from build123d import *
from build123d.topology import SkipClean

# Parameters (mm, degrees)
SKETCH1_W                                       = 111.76
SKETCH1_H                                       = 76.2
BOSS_EXTRUDE1_DEPTH                             = 1.905
FILLET1_R                                       = 2.54
M3_CLEARANCE_HOLE4_D                            = 3.4
CSK_FOR_M3_FLAT_HEAD_MACHINE_SCREW1_D           = 3.4
CSK_FOR_M3_FLAT_HEAD_MACHINE_SCREW1_CSINK_D     = 6.3
CSK_FOR_M3_FLAT_HEAD_MACHINE_SCREW1_CSINK_ANGLE = 90
CSK_FOR_M3_FLAT_HEAD_MACHINE_SCREW2_D           = 3.4
CSK_FOR_M3_FLAT_HEAD_MACHINE_SCREW2_CSINK_D     = 6.3
CSK_FOR_M3_FLAT_HEAD_MACHINE_SCREW2_CSINK_ANGLE = 90
BOSS_EXTRUDE2_START                             = -3.81
SKETCH23_R                                      = 3.15
SKETCH23_R_2                                    = 1.7
BOSS_EXTRUDE2_DEPTH                             = 3.81
SKETCH12_W                                      = 28.355545758
SKETCH12_H                                      = 25.387795591
CUT_EXTRUDE1_DEPTH                              = 68.739947594
M3_CLEARANCE_HOLE1_AT_2_COUNT                   = 2
M3_CLEARANCE_HOLE1_AT_2_PITCH                   = 22.606
FILLET2_R                                       = 2.54


with BuildPart() as part:
    # Sketch1 → Boss-Extrude1 (new, symmetric)
    with BuildSketch(Plane(origin=(0, 0, 0), x_dir=(1, 0, 0), z_dir=(0, 1, 0))):
        Rectangle(SKETCH1_W, SKETCH1_H)
    extrude(amount=BOSS_EXTRUDE1_DEPTH, both=True)

    # Fillet1
    fillet1_edges = [part.edges().sort_by_distance(p)[0] for p in [
        (55.88, 0, 38.1),
        (-55.88, 0, 38.1),
        (-55.88, 0, -38.1),
        (55.88, 0, -38.1),
    ]]
    fillet(fillet1_edges, radius=FILLET1_R)

    # M3 Clearance Hole4 (through all)
    with Locations(Plane(origin=(0, -1.905, 0), x_dir=(-1, 0, 0), z_dir=(0, -1, 0))):
        with Locations((13.38, 34.6), (49.88, 34.6), (50.88, -32.35), (12.38, -32.35)):
            Hole(M3_CLEARANCE_HOLE4_D / 2)

    # CSK for M3 Flat Head Machine Screw1 (through all)
    with Locations(Plane(origin=(0, -1.905, 0), x_dir=(-1, 0, 0), z_dir=(0, -1, 0))):
        with Locations((-51.9557, -16.51), (4.74472, -16.51), (-44.6057, 9.89), (-2.60528, 9.89)):
            CounterSinkHole(CSK_FOR_M3_FLAT_HEAD_MACHINE_SCREW1_D / 2, CSK_FOR_M3_FLAT_HEAD_MACHINE_SCREW1_CSINK_D / 2, counter_sink_angle=CSK_FOR_M3_FLAT_HEAD_MACHINE_SCREW1_CSINK_ANGLE)

    # CSK for M3 Flat Head Machine Screw2 (through all)
    with Locations(Plane(origin=(0, -1.905, 0), x_dir=(-1, 0, 0), z_dir=(0, -1, 0))):
        with Locations((49.88, 23.1), (49.88, -22.4), (13.38, 23.1), (13.38, -22.4)):
            CounterSinkHole(CSK_FOR_M3_FLAT_HEAD_MACHINE_SCREW2_D / 2, CSK_FOR_M3_FLAT_HEAD_MACHINE_SCREW2_CSINK_D / 2, counter_sink_angle=CSK_FOR_M3_FLAT_HEAD_MACHINE_SCREW2_CSINK_ANGLE)

    # Sketch23 → Boss-Extrude2 (add)
    # profile 1 of 2: a face of its own
    with SkipClean():  # the faces are left unmerged after this step: merging them gives an invalid solid
        with BuildSketch(Plane.XZ.offset(1.905).offset(BOSS_EXTRUDE2_START)):
            with Locations((-13.38, 22.4)):
                Circle(SKETCH23_R)
            with Locations(Location((-13.38, 22.4, 0), (0, 0, 270))):
                Circle(SKETCH23_R_2, mode=Mode.SUBTRACT)
        # profile 2 of 2: a face of its own
        with BuildSketch(Plane.XZ.offset(1.905).offset(BOSS_EXTRUDE2_START)):
            with Locations((-49.88, 22.4)):
                Circle(SKETCH23_R)
            with Locations(Location((-49.88, 22.4, 0), (0, 0, 270))):
                Circle(SKETCH23_R_2, mode=Mode.SUBTRACT)
        extrude(amount=BOSS_EXTRUDE2_DEPTH)

    # Sketch12 → Cut-Extrude1 (cut, through all)
    with SkipClean():  # the faces are left unmerged after this step: merging them gives an invalid solid
        with BuildSketch(Plane.XZ.offset(1.905)):
            with Locations((51.007772879, -31.743897796)):
                Rectangle(SKETCH12_W, SKETCH12_H)
        extrude(amount=-CUT_EXTRUDE1_DEPTH, mode=Mode.SUBTRACT)

    # Sketch16 → M3 Clearance Hole1 (revolve, cut)
    with SkipClean():  # the faces are left unmerged after this step: merging them gives an invalid solid
        with BuildSketch(Plane(origin=(30.48, -1.905, 25.4), x_dir=(0, 0, -1), z_dir=(1, 0, 0))):
            Polygon((0, 0), (0, 3.81), (2.85, 3.81), (1.7, 2.66), (1.7, 0), align=None)
        m3_clearance_hole1 = revolve(axis=Axis((30.48, -8.255, 25.4), (0, 1, 0)), mode=Mode.SUBTRACT)

    # M3 Clearance Hole1 at 2: M3 Clearance Hole1 ×2
    with SkipClean():  # the faces are left unmerged after this step: merging them gives an invalid solid
        with Locations(*[(-i * M3_CLEARANCE_HOLE1_AT_2_PITCH, 0, 0) for i in range(1, M3_CLEARANCE_HOLE1_AT_2_COUNT)]):
            add(m3_clearance_hole1, mode=Mode.SUBTRACT)

    # Fillet2
    fillet2_edges = [part.edges().sort_by_distance(p)[0] for p in [
        (36.83, 0, -38.1),
        (55.88, 0, -19.05),
        (36.83, 0, -19.05),
    ]]
    fillet(fillet2_edges, radius=FILLET2_R)


solid = part.part
Here's how the part is built. I have some questions about the finished solid (model axes, mm). A direction names the side the tool comes from. Round coordinates to 2 decimals unless told otherwise and drop trailing zeros. Order: outer loops, then holes, each group sorted by start corner. A loop starts at its lowest first (then second) coordinate and runs counter-clockwise, first axis right, second up. Notation, with made-up numbers: (35, -5) -> (68, -5) arc R29 ccw to (68, 24) -> close; hole circle Ø11 at (20, 40.25). An arc over 180 degrees is marked (long way). Return JSON: item names as keys, results as strings.
Q1. If we section it at D-D on z = 25.4: List the corners of the cut face in (x, y) for me (3 decimals).
Filled sheet:
{"outline": "(-55.88, -1.905) -> (6.174, -1.905) -> (6.174, 0.755) -> (5.024, 1.905) -> (-55.88, 1.905) -> close; (9.574, -1.905) -> (28.78, -1.905) -> (28.78, 0.755) -> (27.63, 1.905) -> (10.724, 1.905) -> (9.574, 0.755) -> close; (32.18, -1.905) -> (55.88, -1.905) -> (55.88, 1.905) -> (33.33, 1.905) -> (32.18, 0.755) -> close"}
Q2. If we section it at C-C on y = -1.2: Give the number of separate pieces and of enclosed holes in the cut face, plus the area to 3 significant figures.
Filled sheet:
{"separate pieces": "1", "enclosed holes": "14", "area": "7,960 mm^2"}
Q3. Which directions (+Z, -Z, +X, -X, +Y, -Y) give clear straight access to the entire face, cutting with the end or side of a thin tool? Please do faces 1 (the flat face through (36.83, 0, -29)), 2 (the cylindrical face through (50.703, 0.742, 15.361)).
Filled sheet:
{"face 1": "-Z, +X, +Y, -Y", "face 2": "+Y, -Y"}
Q4. If we mould it in two halves opening along X, with no side actions, what happens to faces 3 (the flat face through (46, 0, -19.05)), 4 (the cylindrical face through (31.51, -0.59, 26.75)), 5 (the flat face through (-55.88, 0, 0)), 6 (the flat face through (55.88, 0, 10))? For each: released by +X, released by -X, zero draft, split by the parting line, or undercut.
Filled sheet:
{"face 3": "zero draft", "face 4": "undercut", "face 5": "released by -X", "face 6": "released by +X"}
Q5. If we section it at A-A on x = 30.48: List the corners of the cut face in (y, z) for me (3 decimals), plus the area to 3 significant figures.
Filled sheet:
{"outline": "(-1.905, -38.1) -> (1.905, -38.1) -> (1.905, 22.55) -> (0.755, 23.7) -> (-1.905, 23.7) -> close; (-1.905, 27.1) -> (0.755, 27.1) -> (1.905, 28.25) -> (1.905, 38.1) -> (-1.905, 38.1) -> close", "area": "276 mm^2"}
Q6. I need wall thicknesses on line 1 along X through (y, z) = (-1.05, 25.4); line 2 along X through (y, z) = (0.5, 22.4); line 3 along Z through (x, y) = (-5, 0.8). Which ranges of each line are inside material? Lowest first, please. Write a range as from..to.
Filled sheet:
{"line 1": "x = -55.88..6.17, 9.57..28.78, 32.18..55.88", "line 2": "x = -55.88..-51.58, -48.18..-15.08, -11.68..55.88", "line 3": "z = -38.1..14.83, 18.19..38.1"}
Q7. If we section it at B-B on z = 16.51: List the corners of the cut face in (x, y) for me (3 decimals), plus the area to 3 significant figures.
Filled sheet:
{"outline": "(-55.88, -1.905) -> (-7.895, -1.905) -> (-6.445, -0.455) -> (-6.445, 1.905) -> (-55.88, 1.905) -> close; (-3.045, -0.455) -> (-1.595, -1.905) -> (48.806, -1.905) -> (50.256, -0.455) -> (50.256, 1.905) -> (-3.045, 1.905) -> close; (53.656, -0.455) -> (55.106, -1.905) -> (55.88, -1.905) -> (55.88, 1.905) -> (53.656, 1.905) -> close", "area": "396 mm^2"}
Q8. For pin 1 Ø5.5 at (x, z) = (7.874, 25.4) entering from +Y (3 decimals); pin 2 Ø2 at (x, z) = (-49.88, -34.6) entering from +Y; pin 3 Ø4 at (x, z) = (51.96, 16.51) entering from -Y; pin 4 Ø1.1 at (x, y) = (47.5, 1) entering from -Z, each with a flat end and sliding along its axis, tell me the tip position at first contact or that it passes through.
Filled sheet:
{"pin 1": "stops at y = 1.805", "pin 2": "passes through", "pin 3": "stops at y = -0.76", "pin 4": "stops at z = -19.05"}
